Can you work these out from the model? Positions are in its coordinate system, mm. A direction names the side the tool comes from. Give positions to 0.01 mm unless a question says otherwise; leave off trailing zeros. Order: outer loops, then holes, each group sorted by start corner. A loop starts at its lowest first (then second) coordinate and runs counter-clockwise, first axis right, second up.
```python
from build123d import *

# Parameters (mm, degrees)
F0_W     = 101.6
F0_H     = 76.2000028044
F1_DEPTH = 101.6
F2_W     = 50.8
F2_H     = 25.4
F3_DEPTH = 101.6
F4_W     = 50.8
F4_H     = 101.6
F5_DEPTH = 25.4
F6_ANGLE = 90
F7_ANGLE = -90


# Not quite as in the source:
# - a feature names something its author has since deleted; it is built from what else it names


with BuildPart() as f1:
    # F0 (on Top) → F1 (new body)
    with BuildSketch(Plane.XY):
        with Locations((-7.9828569114, 8.4364293143)):
            Rectangle(F0_W, F0_H)
    extrude(amount=F1_DEPTH)

    # F2 (on Top) → F3 (join)
    with BuildSketch(Plane.XY):
        with Locations((-33.3828569114, -42.3635720879)):
            Rectangle(F2_W, F2_H)
    extrude(amount=F3_DEPTH)

    # F4 (on Top) → F5 (join)
    with BuildSketch(Plane.XY):
        with Locations((-33.3828569114, -105.8635720879)):
            Rectangle(F4_W, F4_H)
    extrude(amount=F5_DEPTH)


with BuildPart() as f1_1:
    # F6: moved
    add(f1.part.rotate(Axis((-58.7828569114, -4.2635706857, 101.6), (0, -1, 0)), F6_ANGLE))


with BuildPart() as f1_2:
    # F7: moved
    add(f1_1.part.rotate(Axis((42.8171430886, -156.6635720879, 127), (0, 0, -1)), F7_ANGLE))


solid = f1_2.part
```
1) Suppose I cut it at A-A (z = 131). Please give me the cut outline in (x, y), and give its area (3 significant figures).
2) I'm going to push a flat-ended pin straight in: pin 1 Ø1.5 at (y, z) = (-182.5, 154) entering from +X. Where does the tip first touch, or does it pass through?
3) Which directions (+Z, -Z, +X, -X, +Y, -Y) give clear straight access to the entire face, cutting with the end or side of a thin tool? Please do faces 1 (the face through (-58.783, -220, 127)), 2 (the face through (-84.183, -207, 177)), 3 (the face through (-103, -195, 101.6)).
4) Suppose I cut it at D-D (z = 184). Please give me the cut outline in (x, y), and give its area (3 significant figures).
5) Suppose I cut it at B-B (y = -194). Please give me the cut outline in (x, z).
6) Suppose I cut it at C-C (x = 20.5). Please give me the cut outline in (y, z).
7) If I drill on line 1 (X direction, y = -213, z = 106); line 2 (X direction, y = -164, z = 185); line 3 (Z direction, x = -73.5, y = -162.5), over which ranges is the centre line in solid material (lowest first)?
Results:
1. outline: (-160.38, -258.26) - (-58.78, -258.26) - (-58.78, -182.06) - (42.82, -182.06) - (42.82, -156.66) - (-160.38, -156.66) - close
1. area: 12,900 mm2
2. pin 1: stops at x = -84.18
3. face 1: +Z, -Z, +X, -Y
3. face 2: +Z, +X, +Y, -Y
3. face 3: -Z, +X, -X, +Y, -Y
4. outline: (-160.38, -258.26) - (-84.18, -258.26) - (-84.18, -156.66) - (-160.38, -156.66) - close
4. area: 7,740 mm2
5. outline: (-160.38, 101.6) - (-58.78, 101.6) - (-58.78, 152.4) - (-84.18, 152.4) - (-84.18, 203.2) - (-160.38, 203.2) - close
6. outline: (-182.06, 101.6) - (-156.66, 101.6) - (-156.66, 152.4) - (-182.06, 152.4) - close
7. line 1: x = -160.38 to -58.78
7. line 2: x = -160.38 to -84.18
7. line 3: z = 101.6 to 152.4
